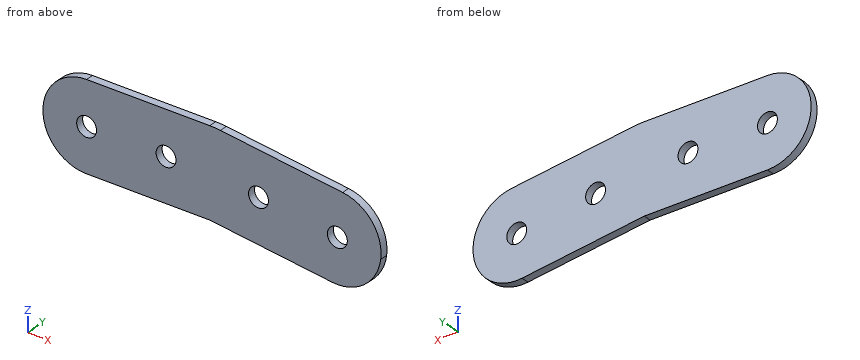
Autodesk Inventor part; units mm, degrees
ref_plane "YZ Plane" through (0, 0, 0) normal (1, 0, 0) x (0, 1, 0)
ref_plane "XZ Plane" through (0, 0, 0) normal (0, 1, 0) x (-1, 0, 0)
ref_plane "XY Plane" through (0, 0, 0) normal (0, 0, 1) x (1, 0, 0)
sketch "Sketch1" plane through (0, 0, 0) normal (0, 1, 0) x (-1, 0, 0)
  line L0 (-11, 0) -> (-42, 0)
  line L1 (-42, 0) -> (-42, -22) construction
  line L2 (-42, -22) -> (-11, -22)
  line L3 (0, -11) -> (0, -11)
  arc A0 (-42, 0) -> (-44.6811, -0.164) centre (-42, -22) ccw
  line L4 (-42, -22) -> (-44.6811, -0.164) construction
  line L5 (-42, -22) -> (-20, -22) construction
  line L6 (-42, -22) -> (-44.6811, -0.164) construction
  line L7 (-44.6811, -0.164) -> (-75.4501, -3.9419)
  line L8 (-85.0275, -16.2005) -> (-85.0275, -16.2005)
  line L9 (-72.7689, -25.7779) -> (-42, -22)
  line L10 (0, 0) -> (-11, 0) construction
  line L11 (-11, 0) -> (-31, 0) construction
  line L12 (-11, 0) -> (-11, -11) construction
  line L13 (-31, 0) -> (-31, -11) construction
  circle A1 centre (-11, -11) radius 2.5
  circle A2 centre (-31, -11) radius 2.5
  line L14 (-44.6811, -0.164) -> (-55.5991, -1.5045) construction
  line L15 (-55.5991, -1.5045) -> (-54.2586, -12.4226) construction
  line L16 (-54.2586, -12.4226) -> (-74.1095, -14.8599) construction
  circle A3 centre (-74.1095, -14.8599) radius 2.5
  circle A4 centre (-54.2586, -12.4226) radius 2.5
  arc A5 (-11, -22) -> (0, -11) centre (-11, -11) ccw
  arc A6 (0, -11) -> (-11, 0) centre (-11, -11) ccw
  arc A7 (-85.0275, -16.2005) -> (-72.7689, -25.7779) centre (-74.1095, -14.8599) ccw
  arc A8 (-75.4501, -3.9419) -> (-85.0275, -16.2005) centre (-74.1095, -14.8599) ccw
  point P0 (0, -22)
  point P1 (-86.3681, -5.2825)
  point P2 (-83.6869, -27.1185)
  dimension "d0" = 42
  dimension "d3" = 97
  dimension "d4" = 42
  dimension "d5" = 11
  dimension "d6" = 20
  dimension "d7" = 22
  dimension "d8" = 11
  dimension "d9" = 11
  dimension "d10" = 5
  dimension "d11" = 5
  dimension "d12" = 11
  dimension "d13" = 11
  dimension "d14" = 90
  dimension "d15" = 20
  dimension "d16" = 5
  dimension "d17" = 5
  dimension "d20" = 11
  dimension "d21" = 11
extrude "Extrusion1" add sketch "Sketch1" along normal blind 2
properties part number "angle bracket"
Here's how the part is built. I have some questions about the finished solid (model axes, mm). Give positions to 0.01 mm unless a question says otherwise; leave off trailing zeros. Write each loop counter-clockwise with the first axis right and the second up, starting at its lowest first coordinate (ties: lowest second). Pieces come first, ordered by that corner, then holes. Notation, with made-up numbers: (54.5, 59) -> (110.5, 59) arc R20 ccw to (110.5, 79) -> close; hole circle Ø6 at (45.5, -8.5). An arc over 180 degrees is marked (long way). Write each question's results on one line, items separated by ' | '.
Item 1: Suppose I cut it at C-C on y = 0.95. Write out the boundary of the cut face in (x, z), plus the area to 3 significant figures.
Output:
outline: (11, -22) -> (42, -22) -> (72.77, -25.78) arc R11 ccw to (75.45, -3.94) -> (44.68, -0.16) arc R22 ccw to (42, 0) -> (11, 0) arc R11 ccw to start; hole circle Ø5 at (11, -11); hole circle Ø5 at (31, -11); hole circle Ø5 at (54.26, -12.42); hole circle Ø5 at (74.11, -14.86) | area: 1,700 mm^2
Item 2: Suppose I cut it at B-B on z = -11. Write out the boundary of the cut face in (x, y).
Output:
outline: (0, 0) -> (8.5, 0) -> (8.5, 2) -> (0, 2) -> close; (13.5, 0) -> (28.5, 0) -> (28.5, 2) -> (13.5, 2) -> close; (33.5, 0) -> (52.2, 0) -> (52.2, 2) -> (33.5, 2) -> close; (56.31, 0) -> (84.41, 0) -> (84.41, 2) -> (56.31, 2) -> close
Item 3: Suppose I cut it at A-A on x = 31. Write out the boundary of the cut face in (y, z).
Output:
outline: (0, -22) -> (2, -22) -> (2, -13.5) -> (0, -13.5) -> close; (0, -8.5) -> (2, -8.5) -> (2, 0) -> (0, 0) -> close
Item 4: If I drill on L1, parallel to X at y = 1.8, z = -13.75; L2, parallel to X at y = 0.55, z = -12; L3, parallel to X at y = 0.15, z = -14, over which ranges is the centre line in solid material (lowest first)?
Output:
L1: x = 0.35 to 52.14, 56.38 to 71.87, 76.35 to 85.05 | L2: x = 0.05 to 8.71, 13.29 to 28.71, 33.29 to 51.79, 56.72 to 84.73 | L3: x = 0.42 to 52.32, 56.2 to 71.76, 76.46 to 85.08
Item 5: Suppose I cut it at D-D on x = 74. Write out the boundary of the cut face in (y, z).
Output:
outline: (0, -25.86) -> (2, -25.86) -> (2, -17.36) -> (0, -17.36) -> close; (0, -12.36) -> (2, -12.36) -> (2, -3.76) -> (0, -3.76) -> close
Item 6: For pin 1 Ø1 at (x, y) = (43.5, 1) entering from -Z, with a flat end and sliding along its axis, tell me the tip position at first contact or that it passes through.
Output:
pin 1: stops at z = -22.25
